The listing builds one solid part. Answer for the finished solid, in the listing's coordinates (mm). A direction names the side the tool comes from. Give positions to 0.01 mm unless a question says otherwise; leave off trailing zeros. Loops run counter-clockwise (first coordinate to the right, second up) from the corner with the lowest first, then second, coordinate; pieces in that order, holes last. Notation, with made-up numbers: (76, 62) - (132, 62) arc R12 cw to (132, 74) - close; hole circle Ø5 at (42.5, -31.75). An arc over 180 degrees is marked (long way). Write item = value, one per line. Start each with the question number.
1) The part is cut by section A-A on x = -8.89. Write down the section's boundary in (y, z) (3 decimals).
2) The mould has two halves that part along X. Classify faces 1 (the flat face through (0, 3, 2)), 2 (the cylindrical face through (-9.85, 3.13, 84.56)), 3 (the flat face through (-21, 7, -152.4)), 4 (the flat face through (-25.4, 13, 2)): +X half, -X half, draft (parallel to the pull), parting line (faces both ways), or undercut.
3) The part is cut by section B-B on z = -88.9. Write down the section's boundary in (x, y) (3 decimals), plus the area to 3 significant figures.
4) Flat-ended cylindrical pins translate along their axes: P1, Ø7, axis at x = -8.89, z = -88.9, coming from the -Y side; P2, Ø5.5, axis at y = 16, z = -40, coming from the +X side; P3, Ø4, axis at x = -12.5, z = 72, coming from the -Y side. Find the tip coordinate at first contact, or state that the pin passes through.
5) The part is cut by section C-C on z = -46. Write down the section's boundary in (x, y), plus the area to 3 significant figures.
6) Consider probe 1 along Z at (x, y) = (-8.89, 4) (3 decimals); probe 2 along Y at (x, z) = (-14, 32.5); probe 3 along X at (y, z) = (3.75, -91). Determine where each line is inside the solid, lowest interval first.
7) The part is cut by section D-D on y = 20.25. Write down the section's boundary in (x, z), plus the area to 3 significant figures.
8) Which of the six approach directions +Z, -Z, +X, -X, +Y, -Y give full straight-line access (tool end or side, diameter ignored) to faces 5 (the flat face through (-19.05, 16, 2)), 6 (the flat face through (-13, 0, 2))?
from build123d import *

# Parameters (mm, degrees)
F1_DEPTH = 152.4
F2_R     = 4.445
F3_DEPTH = 25.4


with BuildPart() as f1:
    # F0 (on Top) → F1 (new body, symmetric)
    with BuildSketch(Plane.XY):
        Polygon((-25.4, 0), (0, 0), (0, 6.35), (-19.05, 6.35), (-19.05, 25.4), (-25.4, 25.4), align=None)
    extrude(amount=F1_DEPTH, both=True)

    # F2 (on face) → F3 (cut)
    with BuildSketch(Plane.XZ):
        with Locations((-8.89, 88.9)):
            Circle(F2_R)
        with Locations((-8.89, -88.9)):
            Circle(F2_R)
    extrude(amount=-F3_DEPTH, mode=Mode.SUBTRACT)


solid = f1.part
Answer below:
q1.outline = (0, -152.4) - (6.35, -152.4) - (6.35, -93.345) - (0, -93.345) - close; (0, -84.455) - (6.35, -84.455) - (6.35, 84.455) - (0, 84.455) - close; (0, 93.345) - (6.35, 93.345) - (6.35, 152.4) - (0, 152.4) - close
q2.face_1 = +X half
q2.face_2 = undercut
q2.face_3 = draft
q2.face_4 = -X half
q3.outline = (-25.4, 0) - (-13.335, 0) - (-13.335, 6.35) - (-19.05, 6.35) - (-19.05, 25.4) - (-25.4, 25.4) - close; (-4.445, 0) - (0, 0) - (0, 6.35) - (-4.445, 6.35) - close
q3.area = 226 mm2
q4.P1 = through
q4.P2 = -19.05
q4.P3 = 0
q5.outline = (-25.4, 0) - (0, 0) - (0, 6.35) - (-19.05, 6.35) - (-19.05, 25.4) - (-25.4, 25.4) - close
q5.area = 282 mm2
q6.probe_1 = -152.4 to -93.345, -84.455 to 84.455, 93.345 to 152.4
q6.probe_2 = 0 to 6.35
q6.probe_3 = -25.4 to -12.81, -4.97 to 0
q7.outline = (-25.4, -152.4) - (-19.05, -152.4) - (-19.05, 152.4) - (-25.4, 152.4) - close
q7.area = 1,940 mm2
q8.face_5 = +Z, -Z, +X, +Y
q8.face_6 = +Z, -Z, +X, -X, -Y
